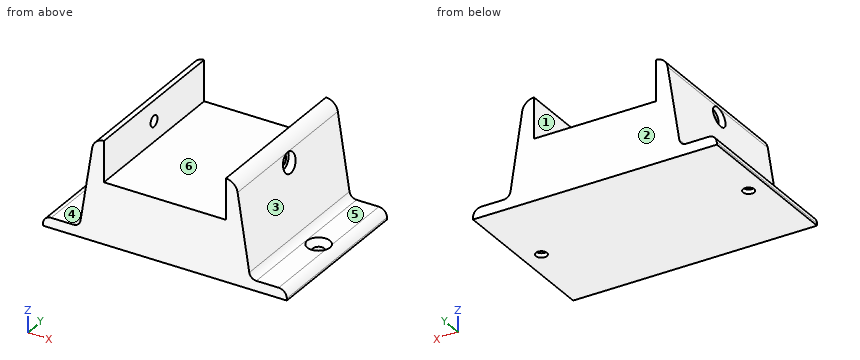
```python
from build123d import *

# Parameters (mm, degrees)
F1_DEPTH              = 80
F10_D                 = 5.5
F10_DEPTH             = 10
F10_CSINK_D           = 11.2
F10_CSINK_ANGLE       = 90
F10_TIP               = 1.6523667023
F10_ON_F3_D           = 5.5
F10_ON_F3_DEPTH       = 10
F10_ON_F3_CSINK_D     = 11.2
F10_ON_F3_CSINK_ANGLE = 90
F10_ON_F3_TIP         = 1.6523667023
F11_D                 = 5.5
F11_DEPTH             = 10
F11_START             = 2.7027778
F11_CBORE_D           = 9.75
F11_CBORE_DEPTH       = 2.5
F11_TIP               = 1.6523667023
F12_D                 = 5.5
F12_DEPTH             = 10
F12_START             = 2.7027778
F12_CBORE_D           = 9.75
F12_CBORE_DEPTH       = 2.5
F12_TIP               = 1.6523667023
F13_T1_DEPTH          = 105.6859695087
F14_R                 = 3.5
F15_T1_DEPTH          = 100


# Not quite as in the source:
# - a fillet or chamfer that OpenCascade refuses, or shapes differently, is made with other operations: its cross-section is extruded or revolved along the edge and cut away or added


with BuildPart() as f1:
    # F0 (on Front) → F1 (new body)
    with BuildSketch(Plane.XZ):
        Polygon((-60, 5), (-60, 0), (60, 0), (60, 5), (42, 5), (35, 50), (30, 50), (30, 30), (-30, 30), (-30, 50), (-35, 50), (-42, 5), align=None)
    extrude(amount=F1_DEPTH)

    # F10
    with Locations(Plane.XY.offset(5)):
        with Locations((-51, -40)):
            CounterSinkHole(F10_D / 2, F10_CSINK_D / 2, depth=F10_DEPTH, counter_sink_angle=F10_CSINK_ANGLE)
            with Locations((0, 0, -(F10_DEPTH + F10_TIP / 2))):  # 118° drill point
                Cone(0, F10_D / 2, F10_TIP, mode=Mode.SUBTRACT)

    # F10 on F3
    with Locations(Plane.XY.offset(5)):
        with Locations((51, -40)):
            CounterSinkHole(F10_ON_F3_D / 2, F10_ON_F3_CSINK_D / 2, depth=F10_ON_F3_DEPTH, counter_sink_angle=F10_ON_F3_CSINK_ANGLE)
            with Locations((0, 0, -(F10_ON_F3_DEPTH + F10_ON_F3_TIP / 2))):  # 118° drill point
                Cone(0, F10_ON_F3_D / 2, F10_ON_F3_TIP, mode=Mode.SUBTRACT)

    # F11
    # its depths count from where the whole tool has entered the part; down to there all is cleared
    with Locations(Plane(origin=(-38.5, 0, 0), x_dir=(0, 1, 0), z_dir=(-1, 0, 0)).offset(-F11_START)):
        with Locations((-40, -40)):
            CounterBoreHole(F11_D / 2, F11_CBORE_D / 2, F11_CBORE_DEPTH, depth=F11_DEPTH)
            with Locations((0, 0, -(F11_DEPTH + F11_TIP / 2))):  # 118° drill point
                Cone(0, F11_D / 2, F11_TIP, mode=Mode.SUBTRACT)

    # F12
    # its depths count from where the whole tool has entered the part; down to there all is cleared
    with Locations(Plane.YZ.offset(38.5).offset(-F12_START)):
        with Locations((-40, 40)):
            CounterBoreHole(F12_D / 2, F12_CBORE_D / 2, F12_CBORE_DEPTH, depth=F12_DEPTH)
            with Locations((0, 0, -(F12_DEPTH + F12_TIP / 2))):  # 118° drill point
                Cone(0, F12_D / 2, F12_TIP, mode=Mode.SUBTRACT)

    # F13: fillet of radius 6 on 2 edges, made by hand

    # F13_s2 → F13_t1 (cut)
    with BuildSketch(Plane.XZ.offset(-12.8429847543)):
        with BuildLine():
            ThreePointArc((-35.7896226953, 44.9238541015), (-33.8164627137, 48.513120963), (-30, 50))
            Line((-30, 50), (-35, 50))
            Line((-35, 50), (-35.7896226953, 44.9238541015))
        make_face()
        with BuildLine():
            ThreePointArc((35.7896226953, 44.9238541015), (33.8164627137, 48.513120963), (30, 50))
            Line((30, 50), (35, 50))
            Line((35, 50), (35.7896226953, 44.9238541015))
        make_face()
    extrude(amount=F13_T1_DEPTH, mode=Mode.SUBTRACT)

    # F14
    f14_edges = [f1.edges().sort_by_distance(p)[0] for p in [
        (-42, -40, 5),
        (42, -40, 5),
    ]]
    fillet(f14_edges, radius=F14_R)

    # F15: fillet of radius 4 on 2 edges, made by hand

    # F15_s2 → F15_t1 (cut)
    with BuildSketch(Plane.XZ.offset(-10)):
        with BuildLine():
            ThreePointArc((-56, 5), (-58.8284271247, 3.8284271247), (-60, 1))
            Line((-60, 1), (-60, 5))
            Line((-60, 5), (-56, 5))
        make_face()
        with BuildLine():
            ThreePointArc((60, 1), (58.8284271247, 3.8284271247), (56, 5))
            Line((56, 5), (60, 5))
            Line((60, 5), (60, 1))
        make_face()
    extrude(amount=F15_T1_DEPTH, mode=Mode.SUBTRACT)


solid = f1.part
```
Source: CAD feature listing. Evaluate the final solid. Frame: model axes, mm. Face numbers are marked on the shaded views. A direction names the side the tool comes from. Give positions to 0.01 mm unless a question says otherwise; leave off trailing zeros. Write each loop counter-clockwise with the first axis right and the second up, starting at its lowest first coordinate (ties: lowest second). Pieces come first, ordered by that corner, then holes.
1. Pull-direction query (X, two-part tool) for the marked faces 1, 2 and 3; classes: +X half, -X half, draft (parallel to the pull), parting line (faces both ways), or undercut.
2. Section query A-A (x = -51). Return the cut outline in (y, z), then the cut area to 3 significant figures.
3. Section query D-D (z = 40). Return the cut outline in (x, y) (3 decimals).
4. Material intervals for line 1 along Y through (x, z) = (34.8, 40) (3 decimals); line 2 along Z through (x, y) = (-47, -18); line 3 along Y through (x, z) = (-31.55, 40), sorted ascending.
5. Access query for the marked faces 4, 5 and 6. Directions: +Z, -Z, +X, -X, +Y, -Y. A direction counts if a zero-diameter tool reaches every point of the face in a straight line with its end or side. Return the directions, or none.
6. First-contact query: pin 1 (5 mm diameter, centred on y = -64, z = 10.5, fed in from -X); pin 2 (9 mm diameter, centred on x = -49, y = -32.5, fed in from +Z); pin 3 (10 mm diameter, centred on y = -55, z = 36.5, fed in from +X). Flat tips, straight axial feed; report the tip coordinate or a pass-through.
7. Section query C-C (y = -12). Return the cut outline in (x, z), then the cut area to 3 significant figures.
Output values:
1. face 1: undercut
1. face 2: draft
1. face 3: +X half
2. outline: (-80, 0) - (-42.75, 0) - (-42.75, 2.15) - (-45.6, 5) - (-80, 5) - close; (-37.25, 0) - (0, 0) - (0, 5) - (-34.4, 5) - (-37.25, 2.15) - close
2. area: 364 mm2
3. outline: (-36.556, -80) - (-30, -80) - (-30, -42.75) - (-33.297, -42.75) - (-33.297, -44.875) - (-36.556, -44.875) - close; (-36.556, -35.125) - (-33.297, -35.125) - (-33.297, -37.25) - (-30, -37.25) - (-30, 0) - (-36.556, 0) - close; (30, -80) - (36.556, -80) - (36.556, -44.875) - (33.297, -44.875) - (33.297, -42.75) - (30, -42.75) - close; (30, -37.25) - (33.297, -37.25) - (33.297, -35.125) - (36.556, -35.125) - (36.556, 0) - (30, 0) - close
4. line 1: y = -80 to -44.875, -35.125 to 0
4. line 2: z = 0 to 5
4. line 3: y = -80 to -42.75, -37.25 to 0
5. face 4: +Z, -X, +Y, -Y
5. face 5: +Z, +X, +Y, -Y
5. face 6: +Z, +Y, -Y
6. pin 1: stops at x = -41.53
6. pin 2: stops at z = 5.04
6. pin 3: stops at x = 37.88
7. outline: (-60, 0) - (60, 0) - (60, 1) arc R4 ccw to (56, 5) - (45, 5) arc R3.5 cw to (41.54, 7.96) - (35.79, 44.92) arc R6 ccw to (30, 50) - (30, 30) - (-30, 30) - (-30, 50) arc R6 ccw to (-35.79, 44.92) - (-41.54, 7.96) arc R3.5 cw to (-45, 5) - (-56, 5) arc R4 ccw to (-60, 1) - close
7. area: 2,850 mm2
